```python
from build123d import *

# Parameters (mm, degrees)
ESQUISSE1_W             = 15
ESQUISSE1_H             = 12
BOSS_EXTRU_1_DEPTH      = 4
ESQUISSE2_W             = 1
ESQUISSE2_H             = 12
BOSS_EXTRU_2_DEPTH      = 4
ESQUISSE3_W             = 13
ESQUISSE3_H             = 1
BOSS_EXTRU_3_DEPTH      = 4
ESQUISSE4_R             = 1.3
ENL_V_MAT_EXTRU_1_DEPTH = 21.808652047
ESQUISSE5_R             = 2.5
ENL_V_MAT_EXTRU_2_DEPTH = 1.5
CHANFREIN1_SIZE         = 1
ESQUISSE6_W             = 11
ESQUISSE6_H             = 8
BOSS_EXTRU_4_DEPTH      = 10
ESQUISSE7_W             = 11.2
ESQUISSE7_H             = 8.2
ENL_V_MAT_EXTRU_3_DEPTH = 10


with BuildPart() as part:
    # Esquisse1 → Boss.-Extru.1 (new body)
    with BuildSketch(Plane(origin=(0, 0, 0), x_dir=(0, 0, -1), z_dir=(1, 0, 0))):
        with Locations((7.5, 6)):
            Rectangle(ESQUISSE1_W, ESQUISSE1_H)
    extrude(amount=BOSS_EXTRU_1_DEPTH)

    # Esquisse2 → Boss.-Extru.2 (add)
    with BuildSketch(Plane(origin=(4, 0, 0), x_dir=(0, 0, -1), z_dir=(1, 0, 0))):
        with Locations((0.5, 6)):
            Rectangle(ESQUISSE2_W, ESQUISSE2_H)
        with Locations((14.5, 6)):
            Rectangle(ESQUISSE2_W, ESQUISSE2_H)
    extrude(amount=BOSS_EXTRU_2_DEPTH)

    # Esquisse3 → Boss.-Extru.3 (add)
    with BuildSketch(Plane(origin=(4, 0, 0), x_dir=(0, 0, -1), z_dir=(1, 0, 0))):
        with Locations((7.5, 11.5)):
            Rectangle(ESQUISSE3_W, ESQUISSE3_H)
        with Locations((7.5, 0.5)):
            Rectangle(ESQUISSE3_W, ESQUISSE3_H)
    extrude(amount=BOSS_EXTRU_3_DEPTH)

    # Esquisse4 → Enlèv. mat.-Extru.1 (cut, through all)
    with BuildSketch(Plane.ZY):
        with Locations((-7.5, 6)):
            Circle(ESQUISSE4_R)
    extrude(amount=-ENL_V_MAT_EXTRU_1_DEPTH, mode=Mode.SUBTRACT)

    # Esquisse5 → Enlèv. mat.-Extru.2 (cut)
    with BuildSketch(Plane.ZY):
        with Locations((-7.5, 6)):
            Circle(ESQUISSE5_R)
    extrude(amount=-ENL_V_MAT_EXTRU_2_DEPTH, mode=Mode.SUBTRACT)

    # Chanfrein1
    chanfrein1_edges = [part.edges().sort_by_distance(p)[0] for p in [
        (0, 6, -10),
    ]]
    chamfer(chanfrein1_edges, length=CHANFREIN1_SIZE)

    # Esquisse6 → Boss.-Extru.4 (add)
    with BuildSketch(Plane.ZY):
        Polygon((-2, 0), (0, 0), (0, 2), (0, 10), (0, 12), (-2, 12), (-13, 12), (-15, 12), (-15, 10), (-15, 2), (-15, 0), (-13, 0), align=None)
        with Locations((-7.5, 6)):
            Rectangle(ESQUISSE6_W, ESQUISSE6_H, mode=Mode.SUBTRACT)
    extrude(amount=BOSS_EXTRU_4_DEPTH)

    # Esquisse7 → Enlèv. mat.-Extru.3 (cut)
    with BuildSketch(Plane.ZY.offset(10)):
        with Locations((-7.5, 6)):
            Rectangle(ESQUISSE7_W, ESQUISSE7_H)
    extrude(amount=-ENL_V_MAT_EXTRU_3_DEPTH, mode=Mode.SUBTRACT)


solid = part.part
```
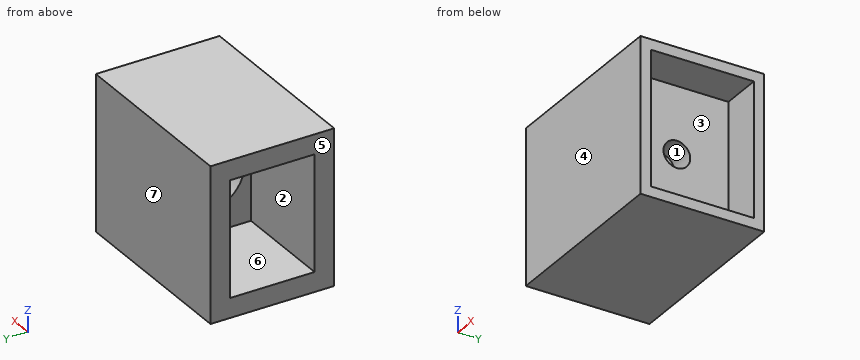
The model under review builds one solid part; all positions refer to its coordinate system, in mm. Face numbers are marked on the shaded views. A direction names the side the tool comes from. Give positions to 0.01 mm unless a question says otherwise; leave off trailing zeros. Write each loop counter-clockwise with the first axis right and the second up, starting at its lowest first coordinate (ties: lowest second). Pieces come first, ordered by that corner, then holes. Notation, with made-up numbers: (-31.5, 3) - (-2.5, 3) arc R6 ccw to (-2.5, 11) - close; hole circle Ø10 at (78, 35). An arc over 180 degrees is marked (long way). Answer in a Markdown table with one row per item. Add a question column.
1. We need section B-B on y = 6. Write out the cut boundary in (x, z).
2. We need section D-D on y = 10.75. Write out the cut boundary in (x, z).
3. We need section A-A on z = -7.5. Write out the cut boundary in (x, y).
4. Wall thickness on line 1 along Z through (x, y) = (4.25, 4); line 2 along Y through (x, z) = (-7, -11); line 3 along Z through (x, y) = (-2, 9.5): over which ranges is each line inside the solid? List them lowest first. Write a range as [from, to].
5. Insertion check: P1, Ø3, axis at y = 6, z = -7.5, coming from the +X side; P2, Ø1.5, axis at x = 1.5, y = 5.5, coming from the +Z side; P3, Ø5.5, axis at y = 7, z = -8, coming from the -X side; P4, Ø2.5, axis at y = 6, z = -7.5, coming from the +X side. Each pin has a flat end and moves straight along its axis. Give the tip position at first contact, or say it passes through.
6. We need section C-C on x = 3.5. Write out the cut boundary in (y, z), then the cut area to 3 significant figures.
7. Draft analysis for pull direction Y (two halves, no side actions). For the marked faces 4, 5, 6 and 7, state which applies: +Y half, -Y half, draft (parallel to the pull), parting line (faces both ways), or undercut.
8. Tool access review of the marked faces 1, 2 and 3: name each direction out of +Z, -Z, +X, -X, +Y, -Y from which nothing blocks a thin tool from reaching the whole face with its end or side.
Ans:
| question | item | result |
|---|---|---|
| 1 | outline | (-10, -15) - (8, -15) - (8, -14) - (4, -14) - (4, -8.8) - (1.5, -8.8) - (1.5, -10) - (1, -10) - (0, -11) - (0, -13.1) - (-10, -13.1) - close; (-10, -1.9) - (0, -1.9) - (0, -4) - (1, -5) - (1.5, -5) - (1.5, -6.2) - (4, -6.2) - (4, -1) - (8, -1) - (8, 0) - (-10, 0) - close |
| 2 | outline | (-10, -15) - (8, -15) - (8, -14) - (4, -14) - (4, -1) - (8, -1) - (8, 0) - (-10, 0) - close |
| 3 | outline | (-10, 0) - (8, 0) - (8, 1) - (4, 1) - (4, 4.7) - (1.5, 4.7) - (1.5, 3.5) - (1, 3.5) - (0, 2.5) - (0, 1.9) - (-10, 1.9) - close; (-10, 10.1) - (0, 10.1) - (0, 9.5) - (1, 8.5) - (1.5, 8.5) - (1.5, 7.3) - (4, 7.3) - (4, 11) - (8, 11) - (8, 12) - (-10, 12) - close |
| 4 | line 1 | z = [-15, -14], [-1, 0] |
| 4 | line 2 | y = [0, 1.9], [10.1, 12] |
| 4 | line 3 | z = [-15, -13.1], [-1.9, 0] |
| 5 | P1 | stops at x = 4 |
| 5 | P2 | stops at z = 0 |
| 5 | P3 | stops at x = 0 |
| 5 | P4 | passes through |
| 6 | outline | (0, -15) - (12, -15) - (12, 0) - (0, 0) - close; hole circle Ø2.6 at (6, -7.5) |
| 6 | area | 175 mm^2 |
| 7 | face 4 | -Y half |
| 7 | face 5 | draft |
| 7 | face 6 | undercut |
| 7 | face 7 | +Y half |
| 8 | face 1 | +X, -X |
| 8 | face 2 | -X |
| 8 | face 3 | +X |
